Source: CAD feature listing. Evaluate the final solid. Frame: model axes, mm. Face numbers are marked on the shaded views. A direction names the side the tool comes from. Round coordinates to 2 decimals unless told otherwise and drop trailing zeros. Order: outer loops, then holes, each group sorted by start corner. A loop starts at its lowest first (then second) coordinate and runs counter-clockwise, first axis right, second up. Notation, with made-up numbers: M 53.25,-36 L 81.25,-36 A23 ccw 81.25,-4 Z; hole C -6,-4 d4. An arc over 180 degrees is marked long. Use CSV: the item, a comma, the result in double quotes. Start each with the question number.
Autodesk Inventor part; units mm, degrees
ref_plane "YZ Plane" through (0, 0, 0) normal (1, 0, 0) x (0, 1, 0)
ref_plane "XZ Plane" through (0, 0, 0) normal (0, 1, 0) x (-1, 0, 0)
ref_plane "XY Plane" through (0, 0, 0) normal (0, 0, 1) x (1, 0, 0)
sketch "Skizze1" plane through (0, 0, 0) normal (1, 0, 0) x (0, 1, 0)
  line L0 (-28, 0) -> (28, 0) construction
  line L1 (0, 35) -> (0, -35) construction
  line L2 (-20, -25) -> (20, -25)
  line L3 (20, -25) -> (20, 25)
  line L4 (20, 25) -> (-20, 25)
  line L5 (-20, 25) -> (-20, -25)
  line L6 (-20, -25) -> (20, 25) construction
  line L7 (20, -25) -> (-20, 25) construction
  point P0 (0, 0)
  dimension "d0" = 40
  dimension "d1" = 50
extrude "Grundkörper" add sketch "Skizze1" along normal mid plane 20
sketch "Skizze2" plane through (10, 0, 0) normal (1, 0, 0) x (0, 0, -1)
  line L0 (-25, 20) -> (-25, -20) construction
  line L1 (0, -28) -> (0, 28) construction
  line L2 (-35, 0) -> (35, 0) construction
  line L3 (-25, -10) -> (5, -10)
  line L4 (5, -10) -> (5, 10)
  line L5 (5, 10) -> (-25, 10)
  line L6 (-25, 10) -> (-25, -10)
  line L7 (25, -20) -> (25, 20) construction
  line L8 (25, -8.4) -> (18, -8.4)
  line L9 (10, -0.4) -> (10, 0.4)
  line L10 (18, 8.4) -> (25, 8.4)
  line L11 (25, -8.4) -> (25, 8.4)
  arc A0 (10, -0.4) -> (18, -8.4) centre (18, -0.4) ccw
  arc A1 (18, 8.4) -> (10, 0.4) centre (18, 0.4) ccw
  point P0 (0, 0)
  dimension "d4" = 30
  dimension "d5" = 20
  dimension "d14" = 15
  dimension "d15" = 16.8
  dimension "d16" = 8
extrude "Ausschnitt" cut sketch "Skizze2" against normal through all
sketch "Skizze4" plane through (-10, -20, -25) normal (0, -1, 0) x (1, 0, 0)
  line L0 (20, 20) -> (0, 20) construction
  line L1 (20, 50) -> (0, 50) construction
  line L2 (10, 60) -> (10, -10)
  line L3 (0, 35) -> (20, 35) construction
  line L4 (0, 0) -> (0, 50) construction
  line L5 (20, 50) -> (20, 0) construction
  point P0 (10, 25)
  point P1 (10, 42.5)
  point P2 (10, 27.5)
  dimension "d19" = 30
  dimension "d20" = 15
  dimension "d21" = 15
hole "DIN7984_M5_Boh" at (0, -20, 17.5) at (0, -20, 2.5) direction (0, 1, 0) diameter 5.5 end up to surface counterbore diameter 10 counterbore depth 3.9
mirror "Spiegeln_DIN7984_M5_Boh" about plane through (0, 0, 0) normal (0, 1, 0) of "DIN7984_M5_Boh"
sketch "Skizze5" plane through (10, -20, -25) normal (0, 0, -1) x (-1, 0, 0)
  line L0 (0, 0) -> (20, 0) construction
  line L1 (20, 11.6) -> (0, 11.6) construction
  line L2 (20, 40) -> (0, 40) construction
  line L3 (0, 28.4) -> (20, 28.4) construction
  line L4 (10, -8) -> (10, 48) construction
  line L5 (-4, 20) -> (24, 20) construction
  line L6 (10, 11.6) -> (10, 0) construction
  point P0 (10, 20)
  point P1 (10, 5.8)
  point P2 (10, 34.2)
  dimension "d29" = 28.4
hole "M5x10" at (0, -14.2, -25) at (0, 14.2, -25) direction (0, 0, 1) diameter 4.134 depth 14.2 tip angle 118 countersink diameter 5 countersink angle 90
chamfer "Fase_Allgemein" distance 4 angle 45 4 edges at (10, -20, 0) (-10, -20, 0) (10, 20, 0) (-10, 20, 0)
chamfer "Fase" distance 0.5 angle 45 15 edges at (10, -6.0569, -12.3431) (10, 0, -10) (10, 6.0569, -12.3431) (10, 8.4, -21.5) (10, -8.4, -21.5) (-10, 6.0569, -12.3431) (-10, 0, -10) (-10, -6.0569, -12.3431) (-10, -8.4, -21.5) (-10, 8.4, -21.5) (-10, 0, -5) (-10, 10, 10) (10, -10, 10) (10, 0, -5) (10, 10, 10)
equation "\"d20\" = 0.5 * d19"
properties part number "200-50-WHEEL-CONNECTOR-01" material "Aluminium 6061"
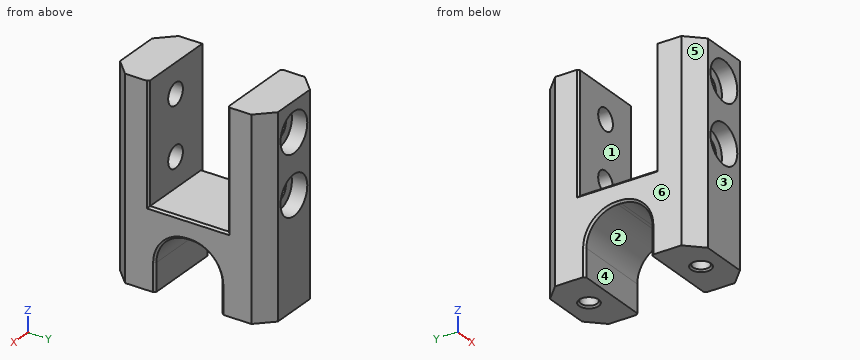
(1) Contact query for flat-ended pins moving along their axis: P1, Ø1.5, axis at x = 8, z = 6, coming from the +Y side; P2, Ø5, axis at x = 0.5, z = 4.5, coming from the +Y side; P3, Ø8, axis at x = 0, z = 17.5, coming from the -Y side. Output: stop coordinate, or through.
(2) Reachability of the marked faces 1, 2 and 3 from +Z, -Z, +X, -X, +Y, -Y: full face, straight path, thin tool, end or side. Return the list, or none.
(3) Line query: line 1 along Z through (x, y) = (0, 11); line 2 along Z through (x, y) = (0, 17.45). Output: solid intervals per line, ascending.
(4) Section C-C on x = 7. Return loops of the section in (y, z), plus the area to 3 significant figures.
(5) Draft query along Y for the marked faces 4, 5 and 6. Return one class per face: pulls with the +Y half, pulls with the -Y half, needs draft (parallel to the pull), parting line crosses it, or undercut.
(6) Section B-B on y = -18. Return loops of the section in (x, z).
(7) Section A-A on z = 2.5. Give the number of separate pieces and of enclosed holes in the cut face, plus the area to 3 significant figures.
Results below:
1,P1,"stops at y = 18.75"
1,P2,"stops at y = 16.1"
1,P3,"stops at y = -16.1"
2,face 1,"+Z, +X, -X"
2,face 2,"-Z, +X, -X"
2,face 3,"+Z, -Z, +X, -X, -Y"
3,line 1,"z = -25 to -0.25, 5.25 to 14.75, 20.25 to 25"
3,line 2,"z = -25 to -2.5, 7.5 to 12.5, 22.5 to 25"
4,outline,"M -19,-25 L -8.4,-25 L -8.4,-18 A8 cw -0.4,-10 L 0.4,-10 A8 cw 8.4,-18 L 8.4,-25 L 19,-25 L 19,25 L 10,25 L 10,-5 L -10,-5 L -10,25 L -19,25 Z"
4,area,"1,080 mm2"
5,face 4,"undercut"
5,face 5,"pulls with the -Y half"
5,face 6,"needs draft"
6,outline,"M -8,-25 L 8,-25 L 8,25 L -8,25 Z; hole C 0,2.5 d10; hole C 0,17.5 d10"
7,separate pieces,"4"
7,enclosed holes,"0"
7,area,"223 mm2"
